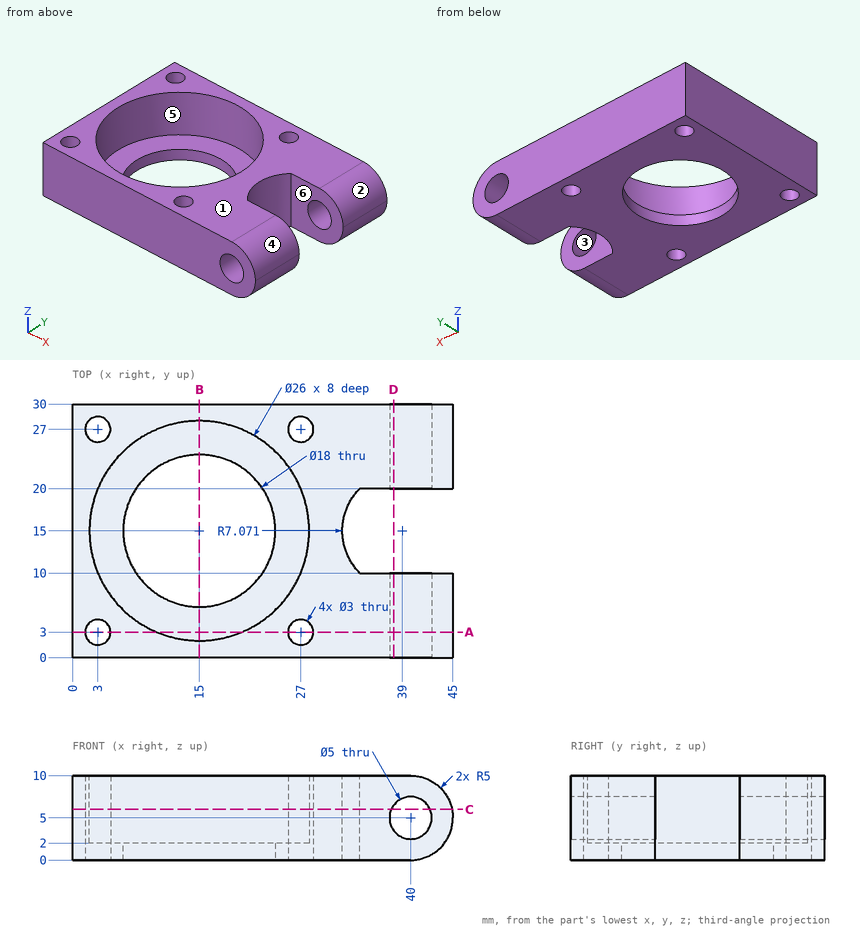
Could you check a few things on this drawing? It's one solid part, dimensions in mm from its lowest x, y, z. A direction names the side the tool comes from. Give positions to 0.01 mm unless a question says otherwise; leave off trailing zeros. Loops run counter-clockwise (first coordinate to the right, second up) from the corner with the lowest first, then second, coordinate; pieces in that order, holes last. Notation, with made-up numbers: (68.5, 27) -> (102.5, 27) arc R26 cw to (102.5, 62) -> close; hole circle Ø5 at (-10, 20). An arc over 180 degrees is marked (long way). Answer as CSV lines item,"result". Start each with the question number.
(1) If we section it at D-D on x = 38: Write out the boundary of the cut face in (y, z).
(2) If we section it at A-A on y = 3: Count the separate pieces of the cut face and the enclosed holes in it, then the cut area to 3 significant figures.
(3) If we section it at C-C on z = 6: Write out the boundary of the cut face in (x, y).
(4) I'm going to push a flat-ended pin straight in: pin 1 Ø2.5 at (x, y) = (3, 3) entering from +Z. Where does the tip first touch, or does it pass through?
(5) I need wall thicknesses on probe 1 along Y at (x, z) = (3, 5); probe 2 along X at (y, z) = (5.25, 5); probe 3 along Y at (x, z) = (4, 7.25). Which ranges of each line are inside material? Lowest first, please.
(6) Which directions (+Z, -Z, +X, -X, +Y, -Y) give clear straight access to the entire face, cutting with the end or side of a thin tool? Please do the marked faces 4, 5 and 6.
(7) If we section it at B-B on x = 15: Write out the boundary of the cut face in (y, z).
(8) We'd pull the mould along X, two halves only. Please class the marked faces 1, 2 and 3: released by +X, released by -X, zero draft, split by the parting line, or undercut.
Computed:
1,outline,"(0, 0) -> (10, 0) -> (10, 3.5) -> (0, 3.5) -> close; (0, 6.5) -> (10, 6.5) -> (10, 10) -> (0, 10) -> close; (20, 0) -> (30, 0) -> (30, 3.5) -> (20, 3.5) -> close; (20, 6.5) -> (30, 6.5) -> (30, 10) -> (20, 10) -> close"
2,separate pieces,"3"
2,enclosed holes,"1"
2,area,"280 mm2"
3,outline,"(0, 0) -> (37.71, 0) -> (37.71, 10) -> (34, 10) arc R7.07 cw to (34, 20) -> (37.71, 20) -> (37.71, 30) -> (0, 30) -> close; (42.29, 0) -> (44.9, 0) -> (44.9, 10) -> (42.29, 10) -> close; (42.29, 20) -> (44.9, 20) -> (44.9, 30) -> (42.29, 30) -> close; hole circle Ø3 at (3, 3); hole circle Ø3 at (3, 27); hole circle Ø26 at (15, 15); hole circle Ø3 at (27, 3); hole circle Ø3 at (27, 27)"
4,pin 1,"passes through"
5,probe 1,"y = 0 to 1.5, 4.5 to 10, 20 to 25.5, 28.5 to 30"
5,probe 2,"x = 0 to 6.4, 23.6 to 37.5, 42.5 to 45"
5,probe 3,"y = 0 to 1.88, 4.12 to 8.07, 21.93 to 25.88, 28.12 to 30"
6,face 4,"+Z, +X, +Y, -Y"
6,face 5,"+Z"
6,face 6,"+Z, -Z, +X"
7,outline,"(0, 0) -> (6, 0) -> (6, 2) -> (2, 2) -> (2, 10) -> (0, 10) -> close; (24, 0) -> (30, 0) -> (30, 10) -> (28, 10) -> (28, 2) -> (24, 2) -> close"
8,face 1,"zero draft"
8,face 2,"released by +X"
8,face 3,"undercut"
